Source: three-view drawing plus pictorial views. Frame: mm from the lowest corner of the part. A direction names the side the tool comes from. Round coordinates to 2 decimals unless told otherwise and drop trailing zeros. Order: outer loops, then holes, each group sorted by start corner. A loop starts at its lowest first (then second) coordinate and runs counter-clockwise, first axis right, second up. Notation, with made-up numbers: (86.5, 6) -> (128.5, 6) arc R26 cw to (128.5, 26) -> close; hole circle Ø2 at (52.25, -7.75). An arc over 180 degrees is marked (long way). Use a Markdown table: item, result.
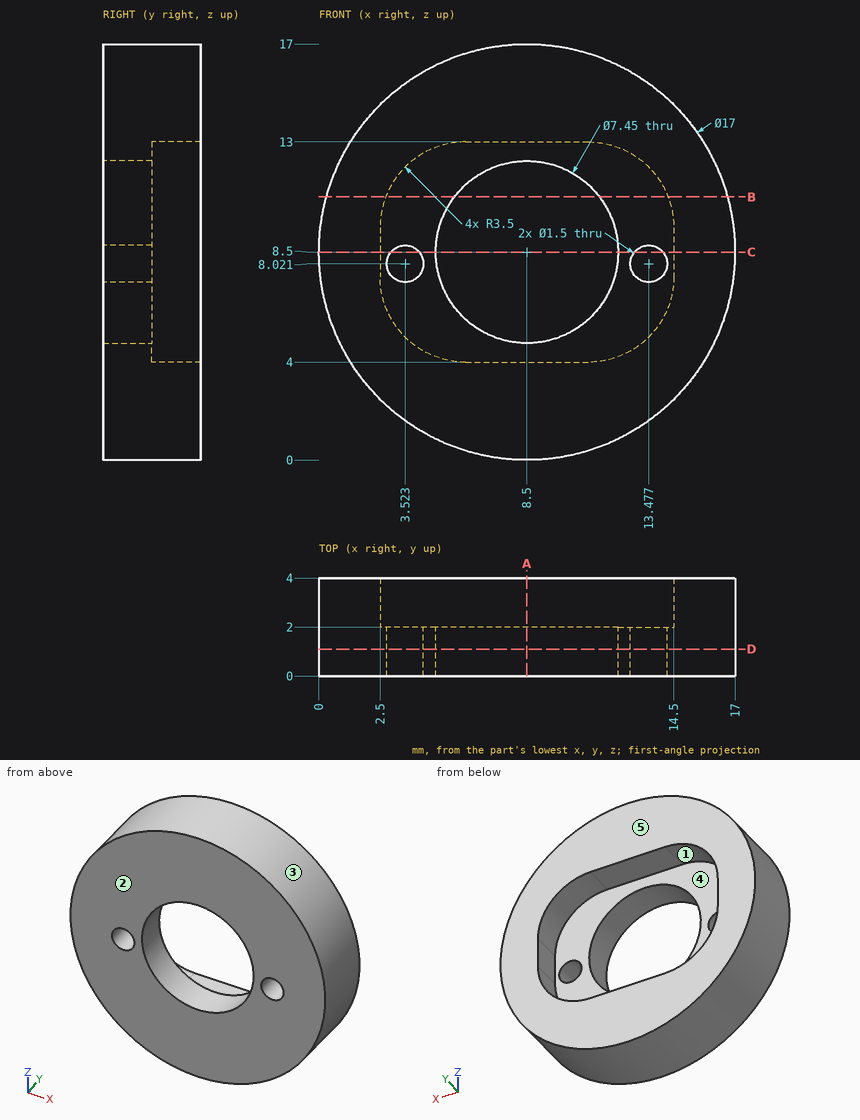
1) Set-up query: the marked faces 4 and 5. Return all of +Z, -Z, +X, -X, +Y, -Y with unobstructed straight access to the full face (end or side cutting, diameter ignored); none if empty.
Results found:
| item | result |
|---|---|
| face 4 | +Y |
| face 5 | +Z, -Z, +X, -X, +Y |
2) Line query: L1, parallel to X at y = 3.3, z = 8.25; L2, parallel to X at y = 1.05, z = 8.5 (1 decimal); L3, parallel to X at y = 1.7, z = 8 (1 decimal). Output: solid intervals per line, ascending. Write a range as [from, to].
Results found:
| item | result |
|---|---|
| L1 | x = [0, 2.5], [14.5, 17] |
| L2 | x = [0, 2.9], [4.1, 4.8], [12.2, 12.9], [14.1, 17] |
| L3 | x = [0, 2.8], [4.3, 4.8], [12.2, 12.7], [14.2, 17] |
3) Cut plane C-C on z = 8.5. Return loops of the section in (x, y) (1 decimal).
Results found:
| item | result |
|---|---|
| outline | (0, 0) -> (2.9, 0) -> (2.9, 2) -> (2.5, 2) -> (2.5, 4) -> (0, 4) -> close; (4.1, 0) -> (4.8, 0) -> (4.8, 2) -> (4.1, 2) -> close; (12.2, 0) -> (12.9, 0) -> (12.9, 2) -> (12.2, 2) -> close; (14.1, 0) -> (17, 0) -> (17, 4) -> (14.5, 4) -> (14.5, 2) -> (14.1, 2) -> close |
4) Cut plane B-B on z = 10.75. Return loops of the section in (x, y).
Results found:
| item | result |
|---|---|
| outline | (0.3, 0) -> (5.53, 0) -> (5.53, 2) -> (2.73, 2) -> (2.73, 4) -> (0.3, 4) -> close; (11.47, 0) -> (16.7, 0) -> (16.7, 4) -> (14.27, 4) -> (14.27, 2) -> (11.47, 2) -> close |
5) Pull-direction query (X, two-part tool) for the marked faces 1, 2 and 3; classes: +X half, -X half, draft (parallel to the pull), parting line (faces both ways), or undercut.
Results found:
| item | result |
|---|---|
| face 1 | undercut |
| face 2 | draft |
| face 3 | parting line |
6) Pin query (flat end, axial travel): pin 1 Ø6 at (x, z) = (8.5, 8.5) entering from +Y; pin 2 Ø2 at (x, y) = (6.5, 2) entering from +Z; pin 3 Ø2 at (y, z) = (1, 12) entering from -X; pin 4 Ø1.5 at (y, z) = (1.5, 5) entering from +X. Return the tip coordinate at first contact, or that it passes through.
Results found:
| item | result |
|---|---|
| pin 1 | passes through |
| pin 2 | stops at z = 16.94 |
| pin 3 | stops at x = 0.38 |
| pin 4 | stops at x = 16.54 |
7) Cut plane D-D on y = 1.1. Count the separate pieces of the cut face and the enclosed holes in it, and give its area (3 significant figures).
Results found:
| item | result |
|---|---|
| separate pieces | 1 |
| enclosed holes | 3 |
| area | 180 mm² |
8) Cut plane A-A on x = 8.5. Return loops of the section in (y, z) (1 decimal).
Results found:
| item | result |
|---|---|
| outline | (0, 0) -> (4, 0) -> (4, 4) -> (2, 4) -> (2, 4.8) -> (0, 4.8) -> close; (0, 12.2) -> (2, 12.2) -> (2, 13) -> (4, 13) -> (4, 17) -> (0, 17) -> close |
